Model file for the job. Use its own axes, mm. A direction names the side the tool comes from. Round coordinates to 2 decimals unless told otherwise and drop trailing zeros. Order: outer loops, then holes, each group sorted by start corner. A loop starts at its lowest first (then second) coordinate and runs counter-clockwise, first axis right, second up. Notation, with made-up numbers: M 11,-6.75 L 63,-6.75 A30 cw 63,22.25 Z; hole C 25.5,25.5 d7. An arc over 180 degrees is marked long. Return JSON: item names as keys, results as strings. Group by question number.
Item 1: Pin check, flat tips, straight feed: pin 1 Ø8 at (y, z) = (4, 35) entering from -X; pin 2 Ø10 at (x, z) = (-16, -7) entering from +Y; pin 3 Ø3 at (x, y) = (-42.5, 12.5) entering from -Z. Stop position of each tip, or through.
Item 2: Slice it at A-A on y = 3.5. Write the cut outline in (x, z) (3 decimals).
Item 3: Pull direction Z, two halves, no side cores. Call faces 4 (the face through (-44, 8, 5)), 5 (the face through (-23, 8, 0)), 6 (the face through (0, 8, 16)), 7 (the face through (-30, 0.99, 2.43)): pulls with the +Z half, pulls with the -Z half, needs draft (parallel to the pull), parting line crosses it, or undercut.
Item 4: Slice it at C-C on z = 16.5. Write the cut outline in (x, y) (3 decimals).
Item 5: Probe line 1 along Z through (x, y) = (-21, 8); line 2 along X through (y, z) = (13.5, 29); line 3 along Z through (x, y) = (-39.5, 8.75) (3 decimals). List the from-to ranges inside material, lowest first.
Item 6: Which spindle directions (+Z, -Z, +X, -X, +Y, -Y) get a long thin tool onto all of the face, cutting with end or side? Do faces 1 (the face through (-45, 8, 16)), 2 (the face through (-33, 2, 17)), 3 (the face through (-15, 0.99, 30.57)). Say none if no direction does.
Item 7: Slice it at B-B on x = -22.5. Write the cut outline in (y, z).
from build123d import *

# Parameters (mm, degrees)
F0_R     = 32.5
F0_W     = 45
F0_H     = 33
F1_DEPTH = 2
F0_R_2   = 0.875
F2_DEPTH = 15
F3_R     = 0.75
F4_R     = 0.75


with BuildPart() as f1:
    # F0 (on Front) → F1 (new body)
    with BuildSketch(Plane.XZ):
        with Locations((-22.5, 16.5)):
            Circle(F0_R)
        with Locations((-22.5, 16.5)):
            Rectangle(F0_W, F0_H, mode=Mode.SUBTRACT)
        with Locations((-22.5, 16.5)):
            Rectangle(F0_W, F0_H)
        with BuildLine():
            Line((-18.5, 32), (-4, 32))
            ThreePointArc((-4, 32), (-1.8786796564, 31.1213203436), (-1, 29))
            Line((-1, 29), (-1, 26.5))
            Line((-1, 26.5), (-1, 6.5))
            Line((-1, 6.5), (-1, 4))
            ThreePointArc((-1, 4), (-1.8786796564, 1.8786796564), (-4, 1))
            Line((-4, 1), (-18.5, 1))
            Line((-18.5, 1), (-26.5, 1))
            Line((-26.5, 1), (-41, 1))
            ThreePointArc((-41, 1), (-43.1213203436, 1.8786796564), (-44, 4))
            Line((-44, 4), (-44, 6.5))
            Line((-44, 6.5), (-44, 26.5))
            Line((-44, 26.5), (-44, 29))
            ThreePointArc((-44, 29), (-43.1213203436, 31.1213203436), (-41, 32))
            Line((-41, 32), (-26.5, 32))
            Line((-26.5, 32), (-18.5, 32))
        make_face(mode=Mode.SUBTRACT)
        with BuildLine():
            ThreePointArc((-1, 29), (-1.8786796564, 31.1213203436), (-4, 32))
            Line((-4, 32), (-18.5, 32))
            ThreePointArc((-18.5, 32), (-14.9644660941, 30.5355339059), (-13.5, 27))
            Line((-13.5, 27), (-13.5, 6))
            ThreePointArc((-13.5, 6), (-14.9644660941, 2.4644660941), (-18.5, 1))
            Line((-18.5, 1), (-4, 1))
            ThreePointArc((-4, 1), (-1.8786796564, 1.8786796564), (-1, 4))
            Line((-1, 4), (-1, 6.5))
            ThreePointArc((-1, 6.5), (-11, 16.5), (-1, 26.5))
            Line((-1, 26.5), (-1, 29))
        make_face()
        with BuildLine():
            ThreePointArc((-31.5, 27), (-30.0355339059, 30.5355339059), (-26.5, 32))
            Line((-26.5, 32), (-41, 32))
            ThreePointArc((-41, 32), (-43.1213203436, 31.1213203436), (-44, 29))
            Line((-44, 29), (-44, 26.5))
            ThreePointArc((-44, 26.5), (-34, 16.5), (-44, 6.5))
            Line((-44, 6.5), (-44, 4))
            ThreePointArc((-44, 4), (-43.1213203436, 1.8786796564), (-41, 1))
            Line((-41, 1), (-26.5, 1))
            ThreePointArc((-26.5, 1), (-30.0355339059, 2.4644660941), (-31.5, 6))
            Line((-31.5, 6), (-31.5, 27))
        make_face()
    extrude(amount=-F1_DEPTH)

    # F0 (on Front) → F2 (join)
    with BuildSketch(Plane.XZ):
        with Locations((-22.5, 16.5)):
            Rectangle(F0_W, F0_H)
        with BuildLine():
            Line((-18.5, 32), (-4, 32))
            ThreePointArc((-4, 32), (-1.8786796564, 31.1213203436), (-1, 29))
            Line((-1, 29), (-1, 26.5))
            Line((-1, 26.5), (-1, 6.5))
            Line((-1, 6.5), (-1, 4))
            ThreePointArc((-1, 4), (-1.8786796564, 1.8786796564), (-4, 1))
            Line((-4, 1), (-18.5, 1))
            Line((-18.5, 1), (-26.5, 1))
            Line((-26.5, 1), (-41, 1))
            ThreePointArc((-41, 1), (-43.1213203436, 1.8786796564), (-44, 4))
            Line((-44, 4), (-44, 6.5))
            Line((-44, 6.5), (-44, 26.5))
            Line((-44, 26.5), (-44, 29))
            ThreePointArc((-44, 29), (-43.1213203436, 31.1213203436), (-41, 32))
            Line((-41, 32), (-26.5, 32))
            Line((-26.5, 32), (-18.5, 32))
        make_face(mode=Mode.SUBTRACT)
        with BuildLine():
            Line((-1, 6.5), (-1, 26.5))
            ThreePointArc((-1, 26.5), (-11, 16.5), (-1, 6.5))
        make_face()
        with Locations((-5.5, 16.5)):
            Circle(F0_R_2, mode=Mode.SUBTRACT)
        with BuildLine():
            ThreePointArc((-44, 6.5), (-34, 16.5), (-44, 26.5))
            Line((-44, 26.5), (-44, 6.5))
        make_face()
        with Locations((-39.5, 16.5)):
            Circle(F0_R_2, mode=Mode.SUBTRACT)
    extrude(amount=-F2_DEPTH)

    # F3
    f3_edges = [f1.edges().sort_by_distance(p)[0] for p in [
        (-55, 0, 16.5),
    ]]
    fillet(f3_edges, radius=F3_R)

    # F4
    f4_edges = [f1.edges().sort_by_distance(p)[0] for p in [
        (0, 15, 16.5),
        (-22.5, 15, 33),
        (-22.5, 15, 0),
        (-45, 15, 16.5),
    ]]
    fillet(f4_edges, radius=F4_R)


solid = f1.part
Output values:
{
 "1": {"pin 1": "x = -51.31", "pin 2": "y = 2", "pin 3": "z = 0"},
 "2": {"outline": "M -45,0 L 0,0 L 0,33 L -45,33 Z; hole M -44,4 A3 ccw -41,1 L -4,1 A3 ccw -1,4 L -1,6.5 A10 cw -1,26.5 L -1,29 A3 ccw -4,32 L -41,32 A3 ccw -44,29 L -44,26.5 A10 cw -44,6.5 Z; hole C -39.5,16.5 d1.75; hole C -5.5,16.5 d1.75"},
 "3": {"face 4": "undercut", "face 5": "pulls with the -Z half", "face 6": "needs draft", "face 7": "undercut"},
 "4": {"outline": "M -55,0.75 A0.75 ccw -54.25,0 L -40.375,0 L -40.375,15 L -44.25,15 A0.75 ccw -45,14.25 L -45,2 L -55,2 Z; M -38.625,0 L -31.5,0 L -31.5,2 L -34,2 L -34,15 L -38.625,15 Z; M -13.5,0 L -6.375,0 L -6.375,15 L -11,15 L -11,2 L -13.5,2 Z; M -4.625,0 L 9.25,0 A0.75 ccw 10,0.75 L 10,2 L 0,2 L 0,14.25 A0.75 ccw -0.75,15 L -4.625,15 Z"},
 "5": {"line 1": "0 to 1, 32 to 33", "line 2": "-45 to -44, -1 to 0", "line 3": "0 to 1, 7.57 to 15.625, 17.375 to 25.43, 32 to 33"},
 "6": {"face 1": "+Z, -Z, -X, +Y", "face 2": "+Y", "face 3": "+Y, -Y"},
 "7": {"outline": "M 0,-15.25 A0.75 ccw 0.75,-16 L 2,-16 L 2,0 L 14.25,0 A0.75 ccw 15,0.75 L 15,1 L 0,1 Z; M 0,32 L 15,32 L 15,32.25 A0.75 ccw 14.25,33 L 2,33 L 2,49 L 0.75,49 A0.75 ccw 0,48.25 Z"}
}
